Answer from the drawing. Dimensions are ordinates in mm from the lowest x, y and z of the part. A direction names the side the tool comes from. Coordinates: 2 decimals unless noted, no trailing zeros. Write each loop counter-clockwise with the first axis right and the second up, starting at its lowest first coordinate (ties: lowest second). Pieces come first, ordered by that corner, then holes.
(1) The part is cut by section C-C, the plane y = 12. Determine the outline of the cut face in (x, z), and give its area (3 significant figures).
(2) The part is cut by section D-D, the plane y = 2.25. Determine the outline of the cut face in (x, z).
(3) The part is cut by section B-B, the plane z = 14.25. Determine the outline of the cut face in (x, y).
(4) The part is cut by section A-A, the plane x = 14.25. Determine the outline of the cut face in (y, z).
(5) Straight lines are drawn through the part: line 1 along Z through (x, y) = (14.25, 3.5); line 2 along X through (y, z) = (19, 14.25); line 3 along Z through (x, y) = (25.25, 1.75). For each, find the intervals that lie inside material, in ascending order.
(6) Determine the mould class of the marked faces 3, 4 and 5 for opening direction Z: pulls with the +Z half, pulls with the -Z half, needs draft (parallel to the pull), parting line crosses it, or undercut.
(7) Given pin 1 (2 mm diameter, centred on y = 15.5, z = 14, fed in from +X); pin 2 (5 mm diameter, centred on y = 10, z = 19, fed in from +X); pin 3 (3.5 mm diameter, centred on x = 14.25, z = 25.25, fed in from +Y), each flat-ended and moving along its own axis, determine where each tip first touches the part or whether it passes through.
(8) Which of the six approach directions +Z, -Z, +X, -X, +Y, -Y give full straight-line access (tool end or side, diameter ignored) to the marked faces 1 and 2?
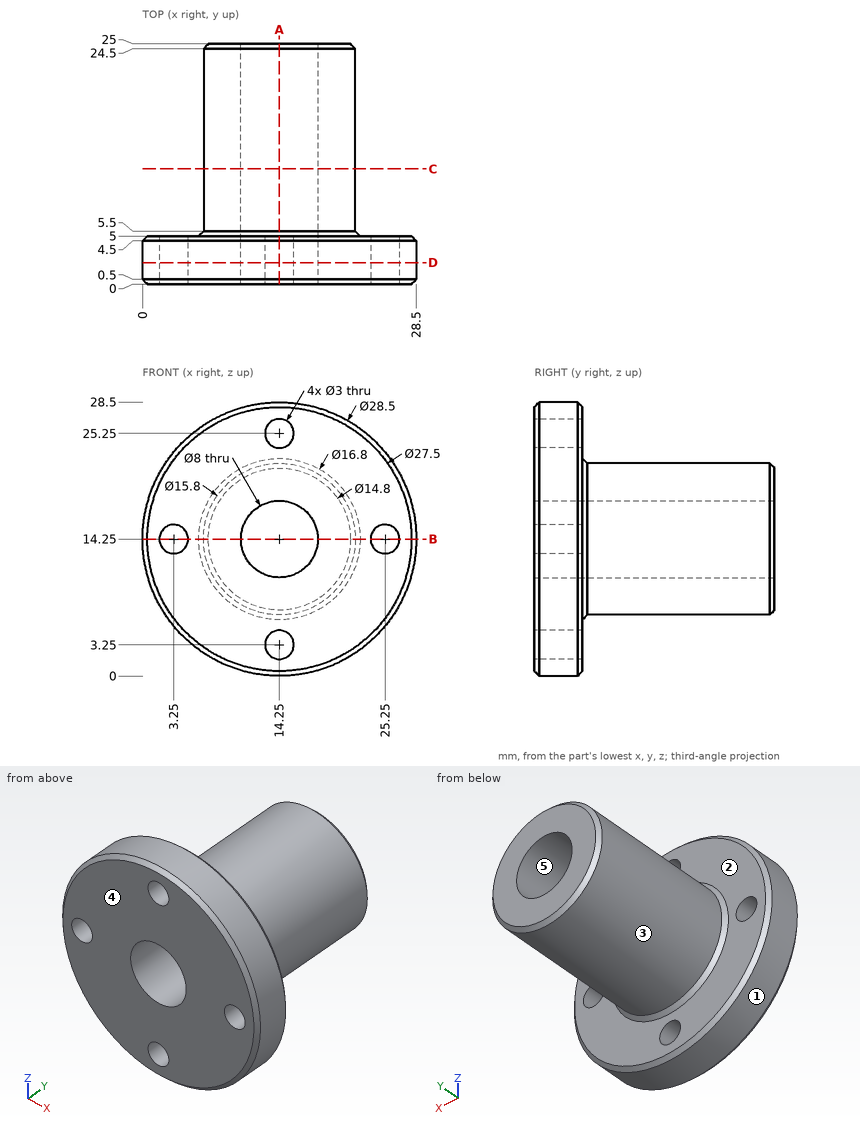
Computed:
1. outline: circle Ø15.8 at (14.25, 14.25); hole circle Ø8 at (14.25, 14.25)
1. area: 146 mm2
2. outline: circle Ø28.5 at (14.25, 14.25); hole circle Ø3 at (3.25, 14.25); hole circle Ø8 at (14.25, 14.25); hole circle Ø3 at (14.25, 3.25); hole circle Ø3 at (14.25, 25.25); hole circle Ø3 at (25.25, 14.25)
3. outline: (0, 0.5) - (0.5, 0) - (1.75, 0) - (1.75, 5) - (0.5, 5) - (0, 4.5) - close; (4.75, 0) - (10.25, 0) - (10.25, 25) - (6.85, 25) - (6.35, 24.5) - (6.35, 5.5) - (5.85, 5) - (4.75, 5) - close; (18.25, 0) - (23.75, 0) - (23.75, 5) - (22.65, 5) - (22.15, 5.5) - (22.15, 24.5) - (21.65, 25) - (18.25, 25) - close; (26.75, 0) - (28, 0) - (28.5, 0.5) - (28.5, 4.5) - (28, 5) - (26.75, 5) - close
4. outline: (0, 0.5) - (0.5, 0) - (4.5, 0) - (5, 0.5) - (5, 1.75) - (0, 1.75) - close; (0, 4.75) - (5, 4.75) - (5, 5.85) - (5.5, 6.35) - (24.5, 6.35) - (25, 6.85) - (25, 10.25) - (0, 10.25) - close; (0, 18.25) - (25, 18.25) - (25, 21.65) - (24.5, 22.15) - (5.5, 22.15) - (5, 22.65) - (5, 23.75) - (0, 23.75) - close; (0, 26.75) - (5, 26.75) - (5, 28) - (4.5, 28.5) - (0.5, 28.5) - (0, 28) - close
5. line 1: z = 0 to 1.75, 4.75 to 10.25, 18.25 to 23.75, 26.75 to 28.5
5. line 2: x = 6.35 to 10.25, 18.25 to 22.15
5. line 3: z = 5.19 to 12.75, 15.75 to 23.31
6. face 3: parting line crosses it
6. face 4: needs draft
6. face 5: undercut
7. pin 1: stops at x = 22.15
7. pin 2: stops at x = 21.82
7. pin 3: stops at y = 5
8. face 1: +Y, -Y
8. face 2: +Y
